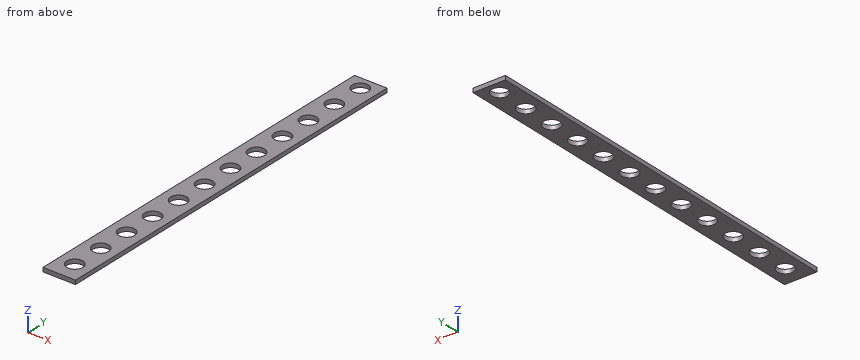
from build123d import *

# Parameters (mm, degrees)
F0_W     = 25.4
F0_H     = 304.8
F1_DEPTH = 3.175
F3_D     = 12.7
F3_DEPTH = 25.4
F3_TIP   = 3.8154649308
F4_D     = 12.7
F4_DEPTH = 25.4
F4_TIP   = 3.8154649308
F5_D     = 12.7
F5_DEPTH = 25.4
F5_TIP   = 3.8154649308
F6_D     = 12.7
F6_DEPTH = 25.4
F6_TIP   = 3.8154649308
F7_D     = 12.7
F7_DEPTH = 25.4
F7_TIP   = 3.8154649308


with BuildPart() as f1:
    # F0 (on Top) → F1 (new body)
    with BuildSketch(Plane.XY):
        Rectangle(F0_W, F0_H)
    extrude(amount=F1_DEPTH)

    # F3
    with Locations(Plane(origin=(0, 0, 0), x_dir=(1, 0, 0), z_dir=(0, 0, -1))):
        with Locations((0, 137.2016693357)):
            Hole(F3_D / 2, depth=F3_DEPTH)
            with Locations((0, 0, -(F3_DEPTH + F3_TIP / 2))):  # 118° drill point
                Cone(0, F3_D / 2, F3_TIP, mode=Mode.SUBTRACT)

    # F4
    with Locations(Plane(origin=(0, 0, 0), x_dir=(1, 0, 0), z_dir=(0, 0, -1))):
        with Locations((0, 111.8016693357)):
            Hole(F4_D / 2, depth=F4_DEPTH)
            with Locations((0, 0, -(F4_DEPTH + F4_TIP / 2))):  # 118° drill point
                Cone(0, F4_D / 2, F4_TIP, mode=Mode.SUBTRACT)

    # F5
    with Locations(Plane(origin=(0, 0, 0), x_dir=(1, 0, 0), z_dir=(0, 0, -1))):
        with Locations((0, 86.4016693357)):
            Hole(F5_D / 2, depth=F5_DEPTH)
            with Locations((0, 0, -(F5_DEPTH + F5_TIP / 2))):  # 118° drill point
                Cone(0, F5_D / 2, F5_TIP, mode=Mode.SUBTRACT)

    # F6
    with Locations(Plane(origin=(0, 0, 0), x_dir=(1, 0, 0), z_dir=(0, 0, -1))):
        with Locations((0, 61.0016693357)):
            Hole(F6_D / 2, depth=F6_DEPTH)
            with Locations((0, 0, -(F6_DEPTH + F6_TIP / 2))):  # 118° drill point
                Cone(0, F6_D / 2, F6_TIP, mode=Mode.SUBTRACT)

    # F7
    with Locations(Plane(origin=(0, 0, 0), x_dir=(1, 0, 0), z_dir=(0, 0, -1))):
        with Locations((0, 35.6016693357), (0, 10.2016693357), (0, -15.1983306643), (0, -40.5983306643), (0, -65.9983306643), (0, -91.3983306643), (0, -116.7983306643), (0, -142.1983306643)):
            Hole(F7_D / 2, depth=F7_DEPTH)
            with Locations((0, 0, -(F7_DEPTH + F7_TIP / 2))):  # 118° drill point
                Cone(0, F7_D / 2, F7_TIP, mode=Mode.SUBTRACT)


solid = f1.part
Can you work these out from the model? Positions are in its coordinate system, mm. Give positions to 0.01 mm unless a question says otherwise; leave off trailing zeros. Loops run counter-clockwise (first coordinate to the right, second up) from the corner with the lowest first, then second, coordinate; pieces in that order, holes last. Notation, with made-up numbers: M 78,42.5 L 94,42.5 A25 cw 94,65.5 Z; hole C 0,-13.5 d4. An arc over 180 degrees is marked long. One line per item, written item: value.
1) Imagine slicing it at A-A on y = -108.5. Write out the boundary of the cut face in (x, z) (3 decimals).
Geometry check:
outline: M -12.7,0 L -5.424,0 L -5.424,3.175 L -12.7,3.175 Z; M 5.424,0 L 12.7,0 L 12.7,3.175 L 5.424,3.175 Z
2) I'm going to push a flat-ended pin straight in: pin 1 (6 mm diameter, centred on x = 2, y = 66.5, fed in from -Z). Where does the tip first touch, or does it pass through?
Geometry check:
pin 1: passes through
3) Please list where these lines run through material, in increasing order: line 1 (X direction, y = -138, z = 0.4); line 2 (X direction, y = -39, z = 1.15).
Geometry check:
line 1: x = -12.7 to -6.3, 6.3 to 12.7
line 2: x = -12.7 to -5.36, 5.36 to 12.7
4) Imagine slicing it at B-B on x = 0. Count the separate pieces of the cut face and the enclosed holes in it, and give its area (3 significant figures).
Geometry check:
separate pieces: 13
enclosed holes: 0
area: 484 mm²
